Geometry: see drawing. Coordinates: mm, zero at the bounding-box minimum. Coordinates: 2 decimals unless noted, no trailing zeros. Loops run counter-clockwise (first coordinate to the right, second up) from the corner with the lowest first, then second, coordinate; pieces in that order, holes last. Notation, with made-up numbers: (23.25, 78) - (69.25, 78) arc R24 ccw to (69.25, 96) - close; hole circle Ø1 at (2.25, 70.25). An arc over 180 degrees is marked (long way). Answer in a Markdown table with one row per item.
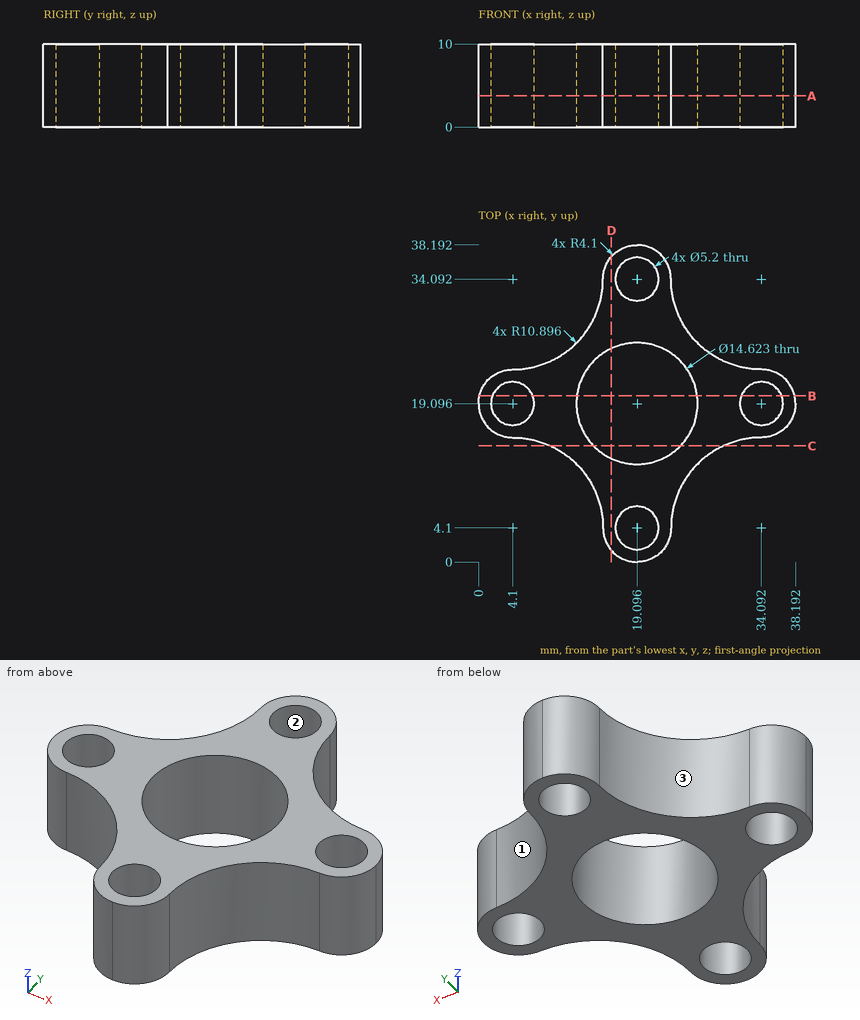
(1) Pull-direction query (X, two-part tool) for the marked faces 1, 2 and 3; classes: pulls with the +X half, pulls with the -X half, needs draft (parallel to the pull), parting line crosses it, or undercut.
Verdict:
| item | result |
|---|---|
| face 1 | pulls with the +X half |
| face 2 | undercut |
| face 3 | pulls with the -X half |
(2) Cut plane C-C on y = 14. Output: boundary loops of the cut face in (x, z), then the cut area to 3 significant figures.
Verdict:
| item | result |
|---|---|
| outline | (8.65, 0) - (13.85, 0) - (13.85, 10) - (8.65, 10) - close; (24.34, 0) - (29.54, 0) - (29.54, 10) - (24.34, 10) - close |
| area | 104 mm² |
(3) Ray query, probe 1 along Y at (x, z) = (19, 5.75) (1 decimal); probe 2 along X at (y, z) = (34, 1) (1 decimal); probe 3 along X at (y, z) = (21, 2) (1 decimal). Return the intervals inside material, ascending.
Verdict:
| item | result |
|---|---|
| probe 1 | y = 0 to 1.5, 6.7 to 11.8, 26.4 to 31.5, 36.7 to 38.2 |
| probe 2 | x = 15 to 16.5, 21.7 to 23.2 |
| probe 3 | x = 0.5 to 2.3, 5.9 to 12, 26.2 to 32.3, 35.9 to 37.7 |
(4) First-contact query: pin 1 Ø4 at (x, y) = (34.09, 19.1) entering from -Z; pin 2 Ø4 at (y, z) = (8, 4) entering from -X; pin 3 Ø3 at (x, z) = (16.5, 5.5) entering from +Y; pin 4 Ø1.5 at (y, z) = (8.5, 7) entering from +X. Flat tips, straight axial feed; report the tip coordinate or a pass-through.
Verdict:
| item | result |
|---|---|
| pin 1 | passes through |
| pin 2 | stops at x = 13.26 |
| pin 3 | stops at y = 38.04 |
| pin 4 | stops at x = 24.49 |
(5) Cut plane A-A on z = 3.75. Output: boundary loops of the cut face in (x, y) (1 decimal), then the cut area to 3 significant figures.
Verdict:
| item | result |
|---|---|
| outline | (4.1, 15) arc R10.9 cw to (15, 4.1) arc R4.1 ccw to (23.2, 4.1) arc R10.9 cw to (34.1, 15) arc R4.1 ccw to (34.1, 23.2) arc R10.9 cw to (23.2, 34.1) arc R4.1 ccw to (15, 34.1) arc R10.9 cw to (4.1, 23.2) arc R4.1 ccw to start; hole circle Ø5.2 at (4.1, 19.1); hole circle Ø14.6 at (19.1, 19.1); hole circle Ø5.2 at (19.1, 4.1); hole circle Ø5.2 at (19.1, 34.1); hole circle Ø5.2 at (34.1, 19.1) |
| area | 379 mm² |
(6) Cut plane D-D on x = 16. Output: boundary loops of the cut face in (y, z).
Verdict:
| item | result |
|---|---|
| outline | (1.41, 0) - (12.47, 0) - (12.47, 10) - (1.41, 10) - close; (25.72, 0) - (36.78, 0) - (36.78, 10) - (25.72, 10) - close |
(7) Cut plane B-B on y = 20. Output: boundary loops of the cut face in (x, z).
Verdict:
| item | result |
|---|---|
| outline | (0.1, 0) - (1.66, 0) - (1.66, 10) - (0.1, 10) - close; (6.54, 0) - (11.84, 0) - (11.84, 10) - (6.54, 10) - close; (26.35, 0) - (31.65, 0) - (31.65, 10) - (26.35, 10) - close; (36.53, 0) - (38.09, 0) - (38.09, 10) - (36.53, 10) - close |
